Model file for the job. Use its own axes, mm. A direction names the side the tool comes from. Coordinates: 2 decimals unless noted, no trailing zeros. Write each loop counter-clockwise with the first axis right and the second up, starting at its lowest first coordinate (ties: lowest second). Pieces come first, ordered by that corner, then holes. Notation, with made-up numbers: M 7.25,27 L 12.25,27 A8 cw 12.25,38 Z; hole C 18.25,-16 d11. An arc over 180 degrees is marked long. One line per question, with ' | ' between items. Start each with the question number.
(1) Wall check: probe 1 along Y at (x, z) = (1.8, -197); probe 2 along Y at (x, z) = (1.8, -189.5); probe 3 along Z at (x, y) = (0.8, -73.5). Give the ranges that are in metal, low to high.
(2) Tool access for faces 4 (the face through (1.61, -26.35, -64.94)), 5 (the face through (0, -40, -135)): list every direction of +Z, -Z, +X, -X, +Y, -Y with a clear straight run to the whole face (end or side of a thin tool).
(3) Flat gauge pins, fed straight in: pin 1 Ø1 at (x, y) = (2, -32.5) entering from +Z; pin 2 Ø1 at (x, z) = (2, -140) entering from -Y; pin 3 Ø1 at (x, y) = (2, -21) entering from +Z. Where does each tip first touch, or does it go through?
(4) Cut at A-A (y = -91.5). Write the cut outline in (x, z) (1 decimal).
(5) Cut at D-D (x = 2.2). Count the separate pieces of the cut face and the enclosed holes in it, plus the area to 3 significant figures.
(6) Two-plate mould, pull along Y, no slides. Class faces 1 (the face through (1.6, 14.4, -139.1)), 2 (the face through (3.175, -40, -135)), 3 (the face through (1.61, -33.69, -57.04)): +Y half, -Y half, draft (parallel to the pull), parting line (faces both ways), or undercut.
(7) Cut at B-B (z = -103). Write the cut outline in (x, y) (3 decimals), plus the area to 3 significant figures.
(8) Cut at C-C (z = -171). Write the cut outline in (x, y) (3 decimals), plus the area to 3 significant figures.
from build123d import *

# Parameters (mm, degrees)
BOSS_EXTRUDE1_DEPTH = 3.175
SKETCH4_W           = 4.7625
SKETCH4_H           = 25.4
CUT_EXTRUDE1_DEPTH  = 318.998242812
BOSS_EXTRUDE2_DEPTH = 3.175
SKETCH8_W           = 4.7625
SKETCH8_H           = 25.4
BOSS_EXTRUDE3_DEPTH = 3.175
CUT_EXTRUDE2_DEPTH  = 3.175
FILLET1_R           = 3.81


with BuildPart() as part:
    # Sketch3 → Boss-Extrude1 (new body)
    with BuildSketch(Plane(origin=(0, 0, 0), x_dir=(0, 0, -1), z_dir=(1, 0, 0))):
        Polygon((0, 0), (274.32, 0), (274.32, -20.32), (279.0825, -20.32), (279.0825, -71.12), (274.32, -71.12), (274.32, -152.4), (0, -20.32), (0, -4.736956919), (-4.7625, -4.736956919), (-4.7625, -2.196956919), (0, -2.196956919), align=None)
    extrude(amount=BOSS_EXTRUDE1_DEPTH)

    # Sketch4 → Cut-Extrude1 (cut, through all)
    with BuildSketch(Plane(origin=(3.175, 0, 0), x_dir=(0, 0, -1), z_dir=(1, 0, 0))):
        with Locations((139.22375, -38.1)):
            Rectangle(SKETCH4_W, SKETCH4_H)
    extrude(amount=-CUT_EXTRUDE1_DEPTH, mode=Mode.SUBTRACT)

    # Sketch7 → Boss-Extrude2 (add)
    with BuildSketch(Plane(origin=(3.175, 0, 0), x_dir=(0, 0, -1), z_dir=(1, 0, 0))):
        Polygon((0, 0), (274.32, 0), (0, 29.21), align=None)
    extrude(amount=-BOSS_EXTRUDE2_DEPTH)

    # Sketch8 → Boss-Extrude3 (add)
    with BuildSketch(Plane(origin=(3.175, 0, 0), x_dir=(0, 0, -1), z_dir=(1, 0, 0))):
        with Locations((-2.38125, 10.503043081)):
            Rectangle(SKETCH8_W, SKETCH8_H)
    extrude(amount=-BOSS_EXTRUDE3_DEPTH)

    # Sketch9 → Cut-Extrude2 (cut)
    with BuildSketch(Plane(origin=(3.175, 0, 0), x_dir=(0, 0, -1), z_dir=(1, 0, 0))):
        Polygon((36.259032566, 12.577289188), (112.24402044, 4.486295109), (58.30952194, -4.892268607), align=None)
        Polygon((12.7, -12.823218546), (12.7, 15.039341432), (41.539031051, -7.808456237), align=None)
        Polygon((33.107422432, -22.165187422), (54.881369429, -18.378958664), (100.799344517, -54.757594352), align=None)
        Polygon((71.651860318, -15.462771034), (124.1425, -6.335277083), (124.1425, -57.048617412), align=None)
        Polygon((171.586571882, -1.832587683), (252.565242685, -10.455316519), (200.256550247, -39.917404217), align=None)
        Polygon((154.305, 0.007579693), (154.305, -65.798926774), (189.093407911, -46.204876971), align=None)
        Polygon((196.79890844, -56.44076101), (154.166437984, -80.452861577), (249.389029774, -126.300776142), align=None)
        Polygon((207.962050776, -50.153288256), (255.27, -23.507794287), (255.27, -112.996536471), align=None)
    extrude(amount=-CUT_EXTRUDE2_DEPTH, mode=Mode.SUBTRACT)

    # Fillet1
    fillet1_edges = [part.edges().sort_by_distance(p)[0] for p in [
        (1.5875, -65.798926774, -154.305),
        (1.5875, -46.204876971, -189.093407911),
        (1.5875, 0.007579693, -154.305),
        (1.5875, -6.335277083, -124.1425),
        (1.5875, -57.048617412, -124.1425),
        (1.5875, -15.462771034, -71.651860318),
        (1.5875, -18.378958664, -54.881369429),
        (1.5875, -54.757594352, -100.799344517),
        (1.5875, -22.165187422, -33.107422432),
        (1.5875, 4.486295109, -112.24402044),
        (1.5875, 12.577289188, -36.259032566),
        (1.5875, -80.452861577, -154.166437984),
        (1.5875, -126.300776142, -249.389029774),
        (1.5875, -56.44076101, -196.79890844),
        (1.5875, -10.455316519, -252.565242685),
        (1.5875, -39.917404217, -200.256550247),
        (1.5875, -1.832587683, -171.586571882),
        (1.5875, -23.507794287, -255.27),
        (1.5875, -112.996536471, -255.27),
        (1.5875, -50.153288256, -207.962050776),
        (1.5875, 15.039341432, -12.7),
        (1.5875, -7.808456237, -41.539031051),
        (1.5875, -12.823218546, -12.7),
    ]]
    fillet(fillet1_edges, radius=FILLET1_R)


solid = part.part
Filled in:
1) probe 1: -115.17 to -101.08, -57.79 to -35.59, -4.54 to 8.23 | probe 2: -111.56 to -97.47, -60.55 to -25.63, -3.74 to 9.03 | probe 3: -274.32 to -255.27, -225.54 to -209.64, -166.51 to -110.45
2) face 4: +X, -X | face 5: +Z, -Z, -X, +Y, -Y
3) pin 1: z = -24.26 | pin 2: y = -87.97 | pin 3: z = -0.37
4) outline: M 0,-274.3 L 3.2,-274.3 L 3.2,-255.3 L 0,-255.3 Z; M 0,-239.1 L 3.2,-239.1 L 3.2,-223.2 L 0,-223.2 Z; M 0,-177.1 L 3.2,-177.1 L 3.2,-147.8 L 0,-147.8 Z
5) separate pieces: 1 | enclosed holes: 9 | area: 18,900 mm²
6) face 1: +Y half | face 2: draft | face 3: undercut
7) outline: M 0,-69.913 L 3.175,-69.913 L 3.175,-40.298 L 0,-40.298 Z; M 0,-10.012 L 3.175,-10.012 L 3.175,18.242 L 0,18.242 Z | area: 184 mm²
8) outline: M 0,-102.653 L 3.175,-102.653 L 3.175,-88.558 L 0,-88.558 Z; M 0,-70.972 L 3.175,-70.972 L 3.175,-56.396 L 0,-56.396 Z; M 0,-22.17 L 3.175,-22.17 L 3.175,11.002 L 0,11.002 Z | area: 196 mm²
